The listing builds one solid part. Answer for the finished solid, in the listing's coordinates (mm). A direction names the side the tool comes from. Coordinates: 2 decimals unless noted, no trailing zeros. Order: outer loops, then holes, each group sorted by start corner. A loop starts at its lowest first (then second) coordinate and runs counter-clockwise, first axis right, second up. Notation, with made-up numbers: (89.5, 76.25) - (93.5, 76.25) arc R21 cw to (93.5, 112.25) - close; hole circle Ø8 at (26.25, 10.5). An arc over 180 degrees is marked (long way). One line per item, written item: value. Start each with the question number.
Autodesk Inventor part; units mm, degrees
ref_plane "YZ Plane" through (0, 0, 0) normal (1, 0, 0) x (0, 1, 0)
ref_plane "XZ Plane" through (0, 0, 0) normal (0, 1, 0) x (-1, 0, 0)
ref_plane "XY Plane" through (0, 0, 0) normal (0, 0, 1) x (1, 0, 0)
sketch "스케치1" plane through (0, 0, 0) normal (0, 0, 1) x (1, 0, 0)
  circle A0 centre (0, 0) radius 22
  dimension "d0" = 44
extrude "돌출1" add sketch "스케치1" along normal blind 2
sketch "스케치2" plane through (0, 0, 2) normal (0, 0, 1) x (1, 0, 0)
  circle A0 centre (0, 0) radius 22
  circle A1 centre (0, 0) radius 19
  circle A2 centre (0, 0) radius 22
  dimension "d7" = 38
extrude "돌출2" add sketch "스케치2" along normal blind 25
sketch "스케치3" plane through (0, 0, 27) normal (0, 0, 1) x (1, 0, 0)
  line L0 (-3, -26.5) -> (3, -26.5)
  line L1 (3, -26.5) -> (3, -20.5)
  line L2 (3, -20.5) -> (-3, -20.5)
  line L3 (-3, -20.5) -> (-3, -26.5)
  circle A0 centre (0, 0) radius 19 construction
  line L4 (0, -19) -> (0, -22) construction
  circle A1 centre (0, 0) radius 22 construction
  line L5 (-1, -24.5) -> (1, -24.5)
  line L6 (1, -24.5) -> (1, -23.5)
  line L7 (1, -23.5) -> (-1, -23.5)
  line L8 (-1, -23.5) -> (-1, -24.5)
  point P0 (0, -20.5)
  point P1 (0, -23.5)
  dimension "d8" = 6
  dimension "d9" = 6
  dimension "d10" = 2
  dimension "d11" = 2
  dimension "d12" = 1
extrude "돌출3" add sketch "스케치3" against normal blind 5
chamfer "모따기1" distance 2 angle 45 1 edges at (0, -22, 22)
pattern_circular "원형 패턴1" count 4 over 360 about axis through (0, 0, 2) along (0, 0, 1) of "돌출3", "모따기1"
properties part number "_3D 인쇄"
(1) For a pull along X with two mould halves and no side action, classify faces 6 (the face through (24.5, 0, 25)), 7 (the face through (0, 23.5, 24)), 8 (the face through (23, 0, 21)), 9 (the face through (-25, 0, 22)) as pulls with the +X half, pulls with the -X half, needs draft (parallel to the pull), parting line crosses it, or undercut.
(2) The part is cut by section D-D on y = 11. Determine the outline of the cut face in (x, z), plus the area to 3 significant figures.
(3) The part is cut by section C-C on z = 14.25. Determine the outline of the cut face in (x, y), plus the area to 3 significant figures.
(4) The part is cut by section A-A on y = 0. Determine the outline of the cut face in (x, z), plus the area to 3 significant figures.
(5) Consider probe 1 along Y at (x, z) = (0, 10.25); probe 2 along Z at (x, y) = (-18, -1); probe 3 along Y at (x, z) = (-22, 25). Determine where each line is inside the solid, lowest interval first.
(6) Flat-ended cylindrical pins translate along their axes: pin 1 Ø0.5 at (x, z) = (-24, 25) entering from +Y; pin 2 Ø1.1 at (y, z) = (24, 25) entering from -X; pin 3 Ø2.5 at (y, z) = (24, 23.5) entering from +X; pin 4 Ø6 at (x, y) = (-21, 18.5) entering from -Z. Find the tip coordinate at first contact, or state that the pin passes through.
(7) For faces 1 (the face through (-3, -24, 24)), 2 (the face through (-24, 3, 24)), 3 (the face through (0, -23.5, 24)), 4 (the face through (8.767, 16.856, 14.325)), 5 (the face through (3, 24, 24)), determine the directions among +Z, -Z, +X, -X, +Y, -Y from which every point of the face is accessible in a straight line to the end or side of a thin tool.
Completed:
1. face 6: undercut
1. face 7: undercut
1. face 8: pulls with the +X half
1. face 9: needs draft
2. outline: (-19.05, 0) - (19.05, 0) - (19.05, 27) - (15.49, 27) - (15.49, 2) - (-15.49, 2) - (-15.49, 27) - (-19.05, 27) - close
2. area: 254 mm2
3. outline: circle Ø44 at (0, 0); hole circle Ø38 at (0, 0)
3. area: 386 mm2
4. outline: (-26.5, 22) - (-24.5, 22) - (-24.5, 27) - (-26.5, 27) - close; (-23.5, 21.5) - (-22, 20) - (-22, 0) - (22, 0) - (22, 20) - (23.5, 21.5) - (23.5, 27) - (19, 27) - (19, 2) - (-19, 2) - (-19, 27) - (-23.5, 27) - close; (24.5, 22) - (26.5, 22) - (26.5, 27) - (24.5, 27) - close
4. area: 277 mm2
5. probe 1: y = -22 to -19, 19 to 22
5. probe 2: z = 0 to 2
5. probe 3: y = -3 to 3
6. pin 1: stops at y = 3
6. pin 2: stops at x = -3
6. pin 3: stops at x = 3
6. pin 4: passes through
7. face 1: +Z, -Z, -X, -Y
7. face 2: +Z, -Z, -X, +Y
7. face 3: +Z, -Z
7. face 4: +Z
7. face 5: +Z, -Z, +X, +Y
